Study the drawing (mm; zero at the part's minimum x, y, z) and answer. Coordinates: 2 decimals unless noted, no trailing zeros. Write each loop counter-clockwise with the first axis right and the second up, starting at its lowest first coordinate (ties: lowest second). Pieces come first, ordered by that corner, then holes. Notation, with made-up numbers: M 27.5,75 L 31.5,75 A21 ccw 31.5,104 Z; hole C 64,34 d9. An arc over 180 degrees is marked long. Answer as a JSON object with one key per item and string values. Group by question number.
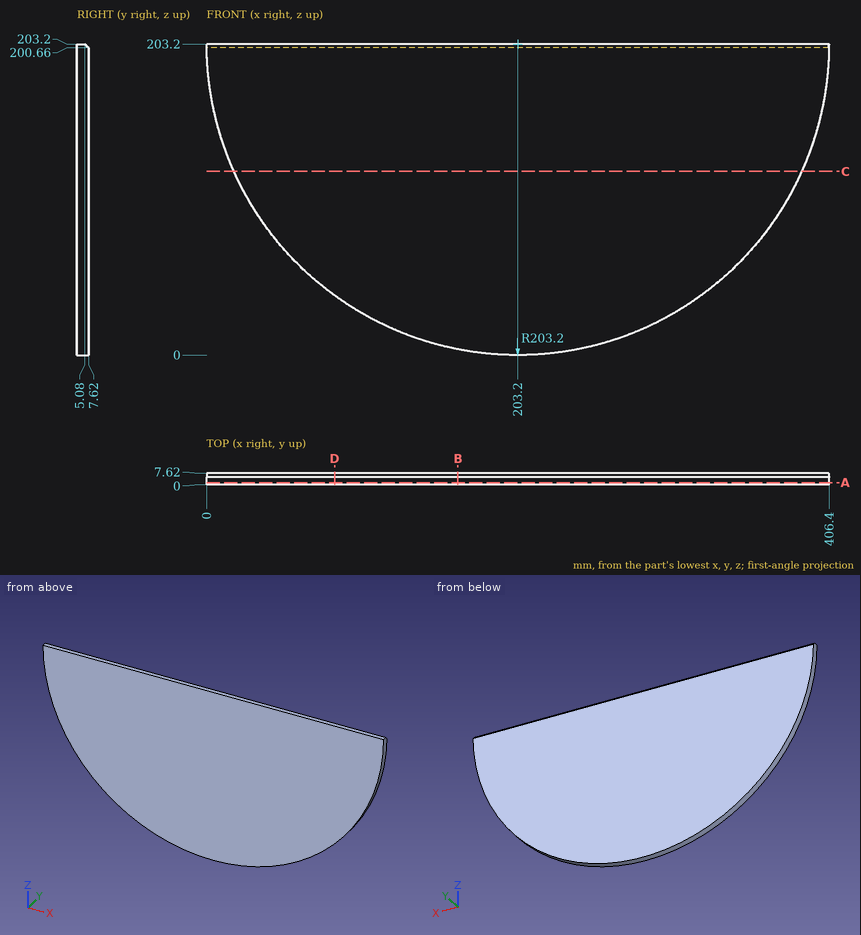
Item 1: A cutting plane is placed at C-C, the plane z = 120. Write down the section's boundary in (x, y).
Item 2: A cutting plane is placed at A-A, the plane y = 1.5. Write down the section's boundary in (x, z), and give its area (3 significant figures).
Item 3: Consider L1, parallel to X at y = 3.75, z = 69.5; L2, parallel to X at y = 3, z = 162.5; L3, parallel to Z at x = 329, y = 1.5. Determine where each line is inside the solid, lowest interval first. Write a range as from..to.
Item 4: Flat-ended cylindrical pins translate along their axes: pin 1 Ø2 at (y, z) = (4, 112.5) entering from +X; pin 2 Ø1.5 at (x, y) = (91, 6) entering from -Z. Find the tip coordinate at first contact, or state that the pin passes through.
Item 5: A cutting plane is placed at D-D, the plane x = 83.5. Write down the section's boundary in (y, z), and give its area (3 significant figures).
Item 6: A cutting plane is placed at B-B, the plane x = 164. Write down the section's boundary in (y, z).
Answer:
{
 "1": {"outline": "M 17.81,0 L 388.59,0 L 388.59,7.62 L 17.81,7.62 Z"},
 "2": {"outline": "M 0,203.2 A203.2 ccw 406.4,203.2 Z", "area": "64,900 mm2"},
 "3": {"L1": "50.18..356.22", "L2": "4.12..402.28", "L3": "43.62..203.2"},
 "4": {"pin 1": "x = 385.53", "pin 2": "z = 33.29"},
 "5": {"outline": "M 0,39 L 7.62,39 L 7.62,200.66 L 5.08,203.2 L 0,203.2 Z", "area": "1,250 mm2"},
 "6": {"outline": "M 0,3.82 L 7.62,3.82 L 7.62,200.66 L 5.08,203.2 L 0,203.2 Z"}
}
